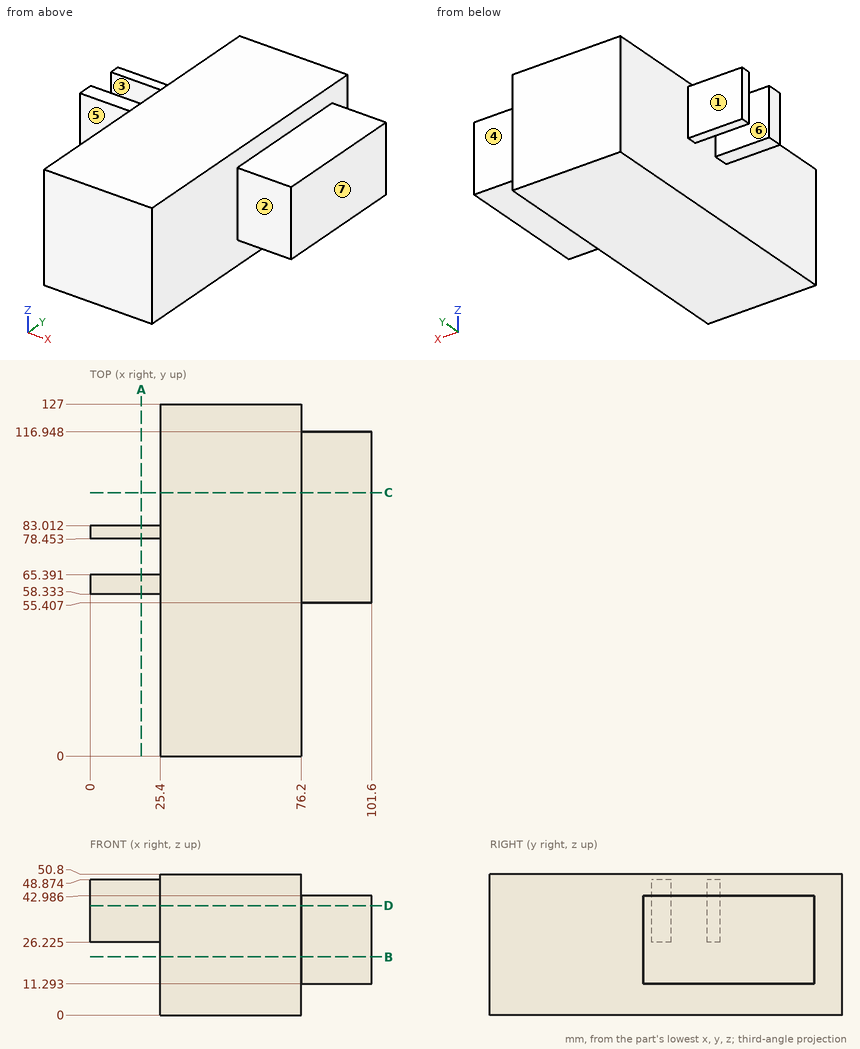
The drawing under review shows one solid part. Ordinate dimensions are in mm from its lowest x, y, z. A direction names the side the tool comes from. Round coordinates to 2 decimals unless told otherwise and drop trailing zeros. Write each loop counter-clockwise with the first axis right and the second up, starting at its lowest first coordinate (ties: lowest second). Pieces come first, ordered by that corner, then holes.
(1) We need section C-C on y = 95. Give the boundary of the cut face in (x, z) (1 decimal).
(2) We need section A-A on x = 18.5. Give the boundary of the cut face in (y, z) (1 decimal), and give its area (3 significant figures).
(3) Wall thickness on L1, parallel to Y at x = 17.5, z = 29; L2, parallel to X at y = 57.5, z = 7.5; L3, parallel to Y at x = 78, z = 29.5: over which ranges is each line inside the solid? List them lowest first.
(4) Mouldability with a two-part tool opening along Y and no side actions: class the marked faces 4, 5, 6 and 7 as +Y half, -Y half, draft (parallel to the pull), parting line (faces both ways), or undercut.
(5) Machinability: for the marked faces 1, 2 and 3, which of the approach directions +Z, -Z, +X, -X, +Y, -Y give a long, thin tool a straight path to every point of the face, cutting with its end or side? Answer none if there is none.
(6) We need section B-B on z = 21. Give the boundary of the cut face in (x, y).
(7) We need section D-D on z = 39.5. Give the boundary of the cut face in (x, y), and give its area (3 significant figures).
(8) Insertion check: pin 1 (11.5 mm diameter, centred on x = 10, z = 43, fed in from -Y); pin 2 (8 mm diameter, centred on x = 13, y = 61, fed in from -Z) (1 decimal); pin 3 (4 mm diameter, centred on x = 42.5, z = 30, fed in from -Y); pin 4 (18 mm diameter, centred on x = 7.5, z = 42.5, fed in from +Y). Each pin has a flat end and moves straight along its axis. Give the tip position at first contact, or say it passes through.
Findings below:
1. outline: (25.4, 0) - (76.2, 0) - (76.2, 11.3) - (101.6, 11.3) - (101.6, 43) - (76.2, 43) - (76.2, 50.8) - (25.4, 50.8) - close
2. outline: (58.3, 26.2) - (65.4, 26.2) - (65.4, 48.9) - (58.3, 48.9) - close; (78.5, 26.2) - (83, 26.2) - (83, 48.9) - (78.5, 48.9) - close
2. area: 263 mm2
3. L1: y = 58.33 to 65.39, 78.45 to 83.01
3. L2: x = 25.4 to 76.2
3. L3: y = 55.41 to 116.95
4. face 4: +Y half
4. face 5: -Y half
4. face 6: undercut
4. face 7: draft
5. face 1: +Z, -Z, -X, +Y
5. face 2: +Z, -Z, +X, -Y
5. face 3: +Z, -Z, -X
6. outline: (25.4, 0) - (76.2, 0) - (76.2, 55.41) - (101.6, 55.41) - (101.6, 116.95) - (76.2, 116.95) - (76.2, 127) - (25.4, 127) - close
7. outline: (0, 58.33) - (25.4, 58.33) - (25.4, 0) - (76.2, 0) - (76.2, 55.41) - (101.6, 55.41) - (101.6, 116.95) - (76.2, 116.95) - (76.2, 127) - (25.4, 127) - (25.4, 83.01) - (0, 83.01) - (0, 78.45) - (25.4, 78.45) - (25.4, 65.39) - (0, 65.39) - close
7. area: 8,310 mm2
8. pin 1: stops at y = 58.33
8. pin 2: stops at z = 26.2
8. pin 3: stops at y = 0
8. pin 4: stops at y = 83.01
